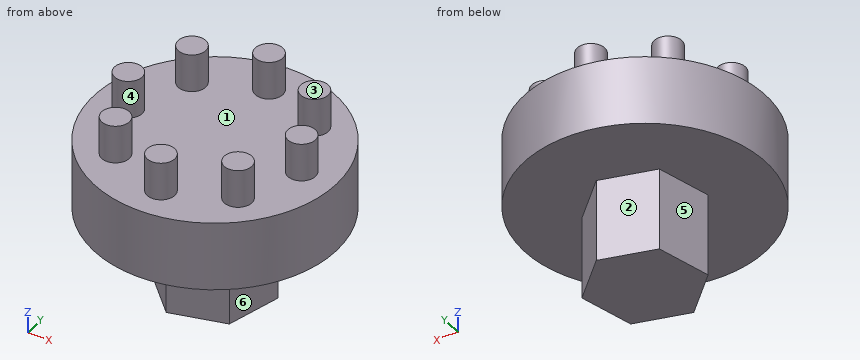
```python
from build123d import *

# Parameters (mm, degrees)
ESQUISSE1_R        = 17.5
BOSS_EXTRU_1_DEPTH = 10
ESQUISSE2_R        = 2
BOSS_EXTRU_2_DEPTH = 5.5
BOSS_EXTRU_3_DEPTH = 12


with BuildPart() as part:
    # Esquisse1 → Boss.-Extru.1 (new body)
    with BuildSketch(Plane.XY):
        Circle(ESQUISSE1_R)
    extrude(amount=BOSS_EXTRU_1_DEPTH)

    # Esquisse2 → Boss.-Extru.2 (add)
    with BuildSketch(Plane.XY.offset(10)):
        with Locations((8.821157095, 8.821157095)):
            Circle(ESQUISSE2_R)
        with Locations((0, 12.475)):
            Circle(ESQUISSE2_R)
        with Locations((12.475, 0)):
            Circle(ESQUISSE2_R)
        with Locations((8.821157095, -8.821157095)):
            Circle(ESQUISSE2_R)
        with Locations((0, -12.475)):
            Circle(ESQUISSE2_R)
        with Locations((-8.821157095, -8.821157095)):
            Circle(ESQUISSE2_R)
        with Locations((-12.475, 0)):
            Circle(ESQUISSE2_R)
        with Locations((-8.821157095, 8.821157095)):
            Circle(ESQUISSE2_R)
    extrude(amount=BOSS_EXTRU_2_DEPTH)

    # Esquisse3 → Boss.-Extru.3 (add)
    with BuildSketch(Plane(origin=(0, 0, 0), x_dir=(-1, 0, 0), z_dir=(0, 0, -1))):
        Polygon((5.662793102, 5.767677835), (-2.163558975, 7.787961601), (-7.826352077, 2.020283765), (-5.662793102, -5.767677835), (2.163558975, -7.787961601), (7.826352077, -2.020283765), align=None)
    extrude(amount=BOSS_EXTRU_3_DEPTH)


solid = part.part
```
Read the model definition and answer for the solid it produces. Units are mm, in the model's axes. Face numbers are marked on the shaded views. A direction names the side the tool comes from. Give positions to 0.01 mm unless a question says otherwise; leave off trailing zeros. Loops run counter-clockwise (first coordinate to the right, second up) from the corner with the lowest first, then second, coordinate; pieces in that order, holes last.
Item 1: The part is cut by section B-B (y = 0). Write down the section's boundary in (x, z) (3 decimals), and give its area (3 significant figures).
Item 2: The part is cut by section A-A (z = 10.75). Write down the section's boundary in (x, y) (3 decimals), and give its area (3 significant figures).
Item 3: Each of these flat-tipped pins is pushed along its axis until it touches: pin 1 Ø12 at (x, z) = (-12.5, 0.5) entering from -Y; pin 2 Ø5 at (y, z) = (10.5, 8.5) entering from -X; pin 3 Ø2 at (y, z) = (-1, 12) entering from +X (3 decimals); pin 4 Ø10 at (x, y) = (6, -5.5) entering from +Z. Where does it stop, or does it pass through?
Item 4: The part is cut by section C-C (x = 11.5). Write down the section's boundary in (y, z), and give its area (3 significant figures).
Item 5: The mould has two halves that part along X. Classify the marked faces 1, 2 and 3: released by +X, released by -X, zero draft, split by the parting line, or undercut.
Item 6: The part is cut by section D-D (z = -6.25). Write down the section's boundary in (x, y), and give its area (3 significant figures).
Item 7: For the marked faces 4, 5 and 6, determine the directions among +Z, -Z, +X, -X, +Y, -Y from which every point of the face is accessible in a straight line to the end or side of a thin tool.
Item 8: Find the intervals of material crossed by line 1 along X through (y, z) = (-9, 11.75); line 2 along Z through (x, y) = (5, -12); line 3 along Z through (x, y) = (9.5, 7), in increasing order.
Taken from the geometry:
1. outline: (-17.5, 0) - (-7.265, 0) - (-7.265, -12) - (7.265, -12) - (7.265, 0) - (17.5, 0) - (17.5, 10) - (14.475, 10) - (14.475, 15.5) - (10.475, 15.5) - (10.475, 10) - (-10.475, 10) - (-10.475, 15.5) - (-14.475, 15.5) - (-14.475, 10) - (-17.5, 10) - close
1. area: 568 mm2
2. outline: circle Ø4 at (-12.475, 0); circle Ø4 at (-8.821, -8.821); circle Ø4 at (-8.821, 8.821); circle Ø4 at (0, -12.475); circle Ø4 at (0, 12.475); circle Ø4 at (8.821, -8.821); circle Ø4 at (8.821, 8.821); circle Ø4 at (12.475, 0)
2. area: 101 mm2
3. pin 1: stops at y = -16.25
3. pin 2: stops at x = -15.56
3. pin 3: stops at x = 14.475
3. pin 4: stops at z = 15.5
4. outline: (-13.19, 0) - (13.19, 0) - (13.19, 10) - (1.75, 10) - (1.75, 15.5) - (-1.75, 15.5) - (-1.75, 10) - (-13.19, 10) - close
4. area: 283 mm2
5. face 1: undercut
5. face 2: released by -X
5. face 3: zero draft
6. outline: (-7.83, -2.02) - (-2.16, -7.79) - (5.66, -5.77) - (7.83, 2.02) - (2.16, 7.79) - (-5.66, 5.77) - close
6. area: 170 mm2
7. face 4: +Z
7. face 5: -Z, -X, +Y
7. face 6: -Z, +X, -Y
8. line 1: x = -10.81 to -6.83, 6.83 to 10.81
8. line 2: z = 0 to 10
8. line 3: z = 0 to 15.5
